from build123d import *

# Parameters (mm, degrees)
SKETCH1_R               = 28.575
BOSS_EXTRUDE1_DEPTH     = 4.7625
SKETCH2_R               = 17.78
CUT_EXTRUDE1_DEPTH      = 5.7625
SKETCH9_R               = 28.575
SKETCH9_R_2             = 17.78
BOSS_EXTRUDE4_DEPTH     = 7.62
SKETCH4_R               = 22.479
SKETCH4_R_2             = 19.304
BOSS_EXTRUDE2_DEPTH     = 5.08
SKETCH5_W               = 6.35
SKETCH5_H               = 50.8
CUT_EXTRUDE3_DEPTH      = 5.08
CUT_EXTRUDE4_DEPTH      = 13.3825
SKETCH10_R              = 19.05
CUT_EXTRUDE5_DEPTH      = 0.59182
SKETCH11_R              = 47.371
SKETCH11_R_2            = 19.05
BOSS_EXTRUDE5_DEPTH     = 3.175
CIRPATTERN1_COUNT       = 6
SKETCH19_R              = 2.4765
CUT_EXTRUDE7_DEPTH      = 21.6375
CIRPATTERN2_COUNT       = 2
CIRPATTERN2_ANGLE       = 25
MIRROR3_COPY_1_SKETCH_R = 2.4765
MIRROR3_COPY_1_DEPTH    = 21.6375
MIRROR4_COPY_1_SKETCH_R = 2.4765
MIRROR4_COPY_1_DEPTH    = 21.6375
MIRROR4_COPY_2_SKETCH_R = 2.4765
MIRROR4_COPY_2_DEPTH    = 21.6375
MIRROR4_COPY_3_SKETCH_R = 2.4765
MIRROR4_COPY_3_DEPTH    = 21.6375


with BuildPart() as part:
    # Sketch1 → Boss-Extrude1 (new body)
    with BuildSketch(Plane.XY):
        Circle(SKETCH1_R)
    extrude(amount=BOSS_EXTRUDE1_DEPTH)

    # Sketch2 → Cut-Extrude1 (cut, through all)
    with BuildSketch(Plane.XY.offset(4.7625)):
        Circle(SKETCH2_R)
    extrude(amount=-CUT_EXTRUDE1_DEPTH, mode=Mode.SUBTRACT)

    # Sketch9 → Boss-Extrude4 (add)
    with BuildSketch(Plane(origin=(0, 0, 0), x_dir=(-1, 0, 0), z_dir=(0, 0, -1))):
        Circle(SKETCH9_R)
        Circle(SKETCH9_R_2, mode=Mode.SUBTRACT)
    extrude(amount=BOSS_EXTRUDE4_DEPTH)

    # Sketch4 → Boss-Extrude2 (add)
    with BuildSketch(Plane.XY.offset(4.7625)):
        Circle(SKETCH4_R)
        Circle(SKETCH4_R_2, mode=Mode.SUBTRACT)
    extrude(amount=BOSS_EXTRUDE2_DEPTH)

    # Sketch5 → Cut-Extrude3 (cut)
    with BuildSketch(Plane.XY.offset(9.8425)):
        Rectangle(SKETCH5_W, SKETCH5_H)
    extrude(amount=-CUT_EXTRUDE3_DEPTH, mode=Mode.SUBTRACT)

    # Sketch7 → Cut-Extrude4 (cut, through all)
    with BuildSketch(Plane.XY.offset(4.7625)):
        with BuildLine():
            ThreePointArc((12.960022594, 28.984484028), (0.147829333, 31.749655848), (-12.689557657, 29.103910845))
            ThreePointArc((-12.689557657, 29.103910845), (-14.330992976, 24.924563995), (-10.151646126, 23.283128676))
            ThreePointArc((-10.151646126, 23.283128676), (0.118263466, 25.399724679), (10.368018075, 23.187587222))
            ThreePointArc((10.368018075, 23.187587222), (14.562468737, 24.790033366), (12.960022594, 28.984484028))
        make_face()
    cut_extrude4 = extrude(amount=-CUT_EXTRUDE4_DEPTH, mode=Mode.SUBTRACT)

    # Mirror1: Cut-Extrude4 across plane
    add(cut_extrude4.mirror(Plane.ZX), mode=Mode.SUBTRACT)

    # Sketch10 → Cut-Extrude5 (cut)
    with BuildSketch(Plane(origin=(0, 0, -7.62), x_dir=(-1, 0, 0), z_dir=(0, 0, -1))):
        Circle(SKETCH10_R)
    extrude(amount=-CUT_EXTRUDE5_DEPTH, mode=Mode.SUBTRACT)

    # Sketch11 → Boss-Extrude5 (add)
    with BuildSketch(Plane(origin=(0, 0, -7.62), x_dir=(-1, 0, 0), z_dir=(0, 0, -1))):
        Circle(SKETCH11_R)
        Circle(SKETCH11_R_2, mode=Mode.SUBTRACT)
    extrude(amount=BOSS_EXTRUDE5_DEPTH)

    # Sketch12 → CSK for #4 Flat Head Socket Cap Screw1 (revolve, cut)
    with BuildSketch(Plane(origin=(-31.75, 0, -10.795), x_dir=(0, 1, 0), z_dir=(1, 0, 0))):
        Polygon((0, 0), (0, 6.060574487), (1.63195, 5.08), (1.63195, 1.848124365), (3.2385, 0), align=None)
    csk_for_4_flat_head_socket_cap_screw1 = revolve(axis=Axis((-31.75, 0, -17.145), (0, 0, 1)), mode=Mode.SUBTRACT)

    # Mirror2: CSK for #4 Flat Head Socket Cap Screw1 across plane
    add(csk_for_4_flat_head_socket_cap_screw1.mirror(Plane(origin=(0, 0, 0), x_dir=(0, 0, 1), z_dir=(1, 0, 0))), mode=Mode.SUBTRACT)

    # Sketch16 → CSK for #4 Flat Head Socket Cap Screw3 (revolve, cut)
    with BuildSketch(Plane(origin=(0, 38.1, -7.62), x_dir=(0, -1, 0), z_dir=(1, 0, 0))):
        Polygon((0, 0), (0, 4.155574487), (1.63195, 3.175), (1.63195, 1.848124365), (3.2385, 0), align=None)
    csk_for_4_flat_head_socket_cap_screw3 = revolve(axis=Axis((0, 38.1, -1.27), (0, 0, -1)), mode=Mode.SUBTRACT)

    # CirPattern1: CSK for #4 Flat Head Socket Cap Screw3 ×6 about axis
    cirpattern1_axis = Axis((0, 0, 0), (0, 0, 1))
    for i in range(1, CIRPATTERN1_COUNT):
        add(csk_for_4_flat_head_socket_cap_screw3.rotate(cirpattern1_axis, i * 360 / CIRPATTERN1_COUNT), mode=Mode.SUBTRACT)

    # Sketch19 → Cut-Extrude7 (cut, through all)
    with BuildSketch(Plane(origin=(0, 0, -10.795), x_dir=(-1, 0, 0), z_dir=(0, 0, -1))):
        with Locations((13.030967461, 35.802288852)):
            Circle(SKETCH19_R)
    cut_extrude7 = extrude(amount=-CUT_EXTRUDE7_DEPTH, mode=Mode.SUBTRACT)

    # CirPattern2: Cut-Extrude7 ×2 about axis
    cirpattern2_axis = Axis((0, 0, -10.795), (0, 0, 1))
    for i in range(1, CIRPATTERN2_COUNT):
        add(cut_extrude7.rotate(cirpattern2_axis, i * CIRPATTERN2_ANGLE / (CIRPATTERN2_COUNT - 1)), mode=Mode.SUBTRACT)

    # Mirror3: Cut-Extrude7 across plane
    add(cut_extrude7.mirror(Plane(origin=(0, 0, 0), x_dir=(0, 0, 1), z_dir=(1, 0, 0))), mode=Mode.SUBTRACT)

    # Mirror3 copy 1 sketch → Mirror3 copy 1 (cut, through all)
    with BuildSketch(Plane(origin=(0, 0, -10.795), x_dir=(0.906307787, -0.422618262, 0), z_dir=(0, 0, -1))):
        with Locations((13.030967461, -35.802288852)):
            Circle(MIRROR3_COPY_1_SKETCH_R)
    extrude(amount=-MIRROR3_COPY_1_DEPTH, mode=Mode.SUBTRACT)

    # Mirror4: Cut-Extrude7 across plane
    add(cut_extrude7.mirror(Plane.ZX), mode=Mode.SUBTRACT)

    # Mirror4 copy 1 sketch → Mirror4 copy 1 (cut, through all)
    with BuildSketch(Plane(origin=(0, 0, -10.795), x_dir=(1, 0, 0), z_dir=(0, 0, -1))):
        with Locations((13.030967461, 35.802288852)):
            Circle(MIRROR4_COPY_1_SKETCH_R)
    extrude(amount=-MIRROR4_COPY_1_DEPTH, mode=Mode.SUBTRACT)

    # Mirror4 copy 2 sketch → Mirror4 copy 2 (cut, through all)
    with BuildSketch(Plane(origin=(0, 0, -10.795), x_dir=(0.906307787, 0.422618262, 0), z_dir=(0, 0, -1))):
        with Locations((13.030967461, 35.802288852)):
            Circle(MIRROR4_COPY_2_SKETCH_R)
    extrude(amount=-MIRROR4_COPY_2_DEPTH, mode=Mode.SUBTRACT)

    # Mirror4 copy 3 sketch → Mirror4 copy 3 (cut, through all)
    with BuildSketch(Plane(origin=(0, 0, -10.795), x_dir=(-0.906307787, 0.422618262, 0), z_dir=(0, 0, -1))):
        with Locations((13.030967461, -35.802288852)):
            Circle(MIRROR4_COPY_3_SKETCH_R)
    extrude(amount=-MIRROR4_COPY_3_DEPTH, mode=Mode.SUBTRACT)


solid = part.part
Input: part model. Units: mm. Frame: model coordinates. A direction names the side the tool comes from. Give positions to 0.01 mm unless a question says otherwise; leave off trailing zeros. Write each loop counter-clockwise with the first axis right and the second up, starting at its lowest first coordinate (ties: lowest second). Pieces come first, ordered by that corner, then holes. Notation, with made-up numbers: (44, -5.5) -> (98, -5.5) arc R13 cw to (98, 11.5) -> close; hole circle Ø1 at (-16.75, -6.75). An arc over 180 degrees is marked (long way). Use one line per item in the form item = value. Start each with the question number.
1) Ray query, probe 1 along Z at (x, y) = (-34, -4) (3 decimals); probe 2 along Y at (x, z) = (4.5, 7.75); probe 3 along X at (y, z) = (2, -3.75). Return the intervals inside material, ascending. Write a range as from..to.
2) Section query D-D on x = 27. Return the cut outline in (y, z) (1 decimal).
3) Set-up query: faces 5 (the cylindrical face through (12.68, 23.08, -1.34)), 6 (the flat face through (-3.175, -21, 7)), 7 (the cylindrical face through (15.12, -11.59, -8.89)). Return all of +Z, -Z, +X, -X, +Y, -Y with unobstructed straight access to the full face (end or side cutting, diameter ignored); none if empty.
4) Section query A-A on x = 0. Count the separate pieces of the cut face and the enclosed holes in it, then the cut area to 3 significant figures.
5) Pin query (flat end, axial travel): pin 1 (5.5 mm diameter, centred on x = 26.94, y = -26.94, fed in from +Z); pin 2 (4.5 mm diameter, centred on x = 13.03, y = -35.8, fed in from -Z); pin 3 (1.5 mm diameter, centred on x = 38, z = -8.5, fed in from -Y); pin 4 (1.6 mm diameter, centred on y = 21, z = 6.5, fed in from +X). Return the tip coordinate at first contact, or that it passes through.
6) Draft query along Y for faces 1 (the cylindrical face through (-24.652, -27.888, -9.23)), 2 (the cylindrical face through (-12.53, 23.22, -1.34)), 3 (the flat face through (-19.3, -3.2, 9.843)), 4 (the cylindrical face through (-28.57, -0.42, -1.34)). Return one class per face: pulls with the +Y half, pulls with the -Y half, needs draft (parallel to the pull), parting line crosses it, or undercut.
7) Section query C-C on z = 3. Return the cut outline in (x, y) (3 decimals).
Outcome:
q1.probe_1 = -10.795..-7.62
q1.probe_2 = -22.02..-18.77, 18.77..22.02
q1.probe_3 = -28.5..-17.67, 17.67..28.5
q2.outline = (-38.9, -10.8) -> (-29.4, -10.8) -> (-29.4, -7.6) -> (-38.9, -7.6) -> close; (-24.5, -10.8) -> (24.5, -10.8) -> (24.5, -7.6) -> (9.4, -7.6) -> (9.4, 4.8) -> (-9.4, 4.8) -> (-9.4, -7.6) -> (-24.5, -7.6) -> close; (29.4, -10.8) -> (38.9, -10.8) -> (38.9, -7.6) -> (29.4, -7.6) -> close
q3.face_5 = +Z, +Y
q3.face_6 = +Z, +Y, -Y
q3.face_7 = -Z
q4.separate_pieces = 4
q4.enclosed_holes = 0
q4.area = 340 mm^2
q5.pin_1 = -7.62
q5.pin_2 = through
q5.pin_3 = -29.27
q5.pin_4 = 9.86
q6.face_1 = undercut
q6.face_2 = pulls with the +Y half
q6.face_3 = needs draft
q6.face_4 = parting line crosses it
q7.outline = (-14.256, -24.765) arc R3.175 cw to (-10.152, -23.283) arc R25.4 ccw to (10.368, -23.188) arc R3.175 cw to (14.486, -24.631) arc R28.575 ccw to (14.486, 24.631) arc R3.175 cw to (10.368, 23.188) arc R25.4 ccw to (-10.152, 23.283) arc R3.175 cw to (-14.256, 24.765) arc R28.575 ccw to start; hole circle Ø35.56 at (0, 0)
